Input: part model. Units: mm. Frame: model coordinates. A direction names the side the tool comes from. Coordinates: 2 decimals unless noted, no trailing zeros. Order: outer loops, then holes, each group sorted by start corner. A loop starts at its lowest first (then second) coordinate and runs counter-clockwise, first axis right, second up. Notation, with made-up numbers: (1, 16.5) -> (9, 16.5) arc R14 cw to (9, 20.5) -> close; hole circle Ø4 at (-35, -7.5). An arc over 180 degrees is marked (long way). One line per question, with ' | ' between items.
```python
from build123d import *

# Parameters (mm, degrees)
SKETCH1_W           = 50
SKETCH1_H           = 60
BOSS_EXTRUDE1_DEPTH = 2.85
SKETCH2_W           = 10
SKETCH2_H           = 2.85
BOSS_EXTRUDE2_DEPTH = 2.85
CUT_EXTRUDE1_DEPTH  = 42.379282256
SKETCH4_R           = 1.425
SKETCH4_W           = 10
SKETCH4_H           = 2.85
CUT_EXTRUDE2_DEPTH  = 42.379282256


with BuildPart() as part:
    # Sketch1 → Boss-Extrude1 (new body)
    with BuildSketch(Plane(origin=(0, 0, 0), x_dir=(1, 0, 0), z_dir=(0, 1, 0))):
        Rectangle(SKETCH1_W, SKETCH1_H)
    extrude(amount=BOSS_EXTRUDE1_DEPTH)

    # Sketch2 → Boss-Extrude2 (add)
    with BuildSketch(Plane(origin=(0, 2.85, 0), x_dir=(1, 0, 0), z_dir=(0, 1, 0))):
        with Locations((-15, 31.425)):
            Rectangle(SKETCH2_W, SKETCH2_H)
        with Locations((15, 31.425)):
            Rectangle(SKETCH2_W, SKETCH2_H)
    boss_extrude2 = extrude(amount=-BOSS_EXTRUDE2_DEPTH)

    # Sketch3 → Cut-Extrude1 (cut, through all)
    with BuildSketch(Plane(origin=(0, 2.85, 0), x_dir=(1, 0, 0), z_dir=(0, 1, 0))):
        Polygon((-4, 26), (-1.7, 26), (-1.7, 30), (1.7, 30), (1.7, 26), (4, 26), (4, 23), (1.7, 23), (1.7, 20), (-1.7, 20), (-1.7, 23), (-4, 23), align=None)
    cut_extrude1 = extrude(amount=-CUT_EXTRUDE1_DEPTH, mode=Mode.SUBTRACT)

    # Mirror1: Boss-Extrude2, Cut-Extrude1 across plane
    add(boss_extrude2.mirror(Plane.XY))
    add(cut_extrude1.mirror(Plane.XY), mode=Mode.SUBTRACT)

    # Sketch4 → Cut-Extrude2 (cut, through all)
    with BuildSketch(Plane(origin=(0, 2.85, 0), x_dir=(1, 0, 0), z_dir=(0, 1, 0))):
        with Locations(Location((0, 0.515, 0), (0, 0, 270))):
            Circle(SKETCH4_R)
        with Locations((-15, 0.515)):
            Rectangle(SKETCH4_W, SKETCH4_H)
        with Locations((15, 0.515)):
            Rectangle(SKETCH4_W, SKETCH4_H)
    extrude(amount=-CUT_EXTRUDE2_DEPTH, mode=Mode.SUBTRACT)


solid = part.part
```
1. Cut plane B-B, the plane z = -21. Return loops of the section in (x, y).
Recorded:
outline: (-25, 0) -> (-1.7, 0) -> (-1.7, 2.85) -> (-25, 2.85) -> close; (1.7, 0) -> (25, 0) -> (25, 2.85) -> (1.7, 2.85) -> close
2. Cut plane D-D, the plane y = 0.9. State how many separate pieces and enclosed holes the cut face has, and give its area (3 significant figures).
Recorded:
separate pieces: 1 | enclosed holes: 3 | area: 2,960 mm^2
3. Mould query, pull axis X, two halves, no side actions, for faces 6 (the face through (-20, 1, 31)), 7 (the face through (-1.7, 1, -28)), 8 (the face through (25, 1, 0)), 9 (the face through (15, 1, 32.85)). Classes: released by +X, released by -X, zero draft, split by the parting line, or undercut.
Recorded:
face 6: released by -X | face 7: undercut | face 8: released by +X | face 9: zero draft
4. Cut plane C-C, the plane z = -1. Return loops of the section in (x, y), and give its area (3 significant figures).
Recorded:
outline: (-25, 0) -> (-20, 0) -> (-20, 2.85) -> (-25, 2.85) -> close; (-10, 0) -> (-1.34, 0) -> (-1.34, 2.85) -> (-10, 2.85) -> close; (1.34, 0) -> (10, 0) -> (10, 2.85) -> (1.34, 2.85) -> close; (20, 0) -> (25, 0) -> (25, 2.85) -> (20, 2.85) -> close | area: 77.9 mm^2
5. Pin query (flat end, axial travel): pin 1 Ø1.2 at (x, y) = (3, 1.5) entering from -Z; pin 2 Ø0.9 at (y, z) = (2, 32) entering from -X; pin 3 Ø0.9 at (x, y) = (0.5, 1.5) entering from -Z. Return the tip coordinate at first contact, or that it passes through.
Recorded:
pin 1: stops at z = -30 | pin 2: stops at x = -20 | pin 3: stops at z = -20
6. Access query for faces 1 (the face through (-25, 1, 0)), 2 (the face through (-20, 1, 0)), 3 (the face through (-20, 1, -31)), 4 (the face through (1.7, 1, -22)), 5 (the face through (0, 1, 20)). Directions: +Z, -Z, +X, -X, +Y, -Y. A direction counts if a zero-diameter tool reaches every point of the face in a straight line with its end or side. Return the directions, or none.
Recorded:
face 1: +Z, -Z, -X, +Y, -Y | face 2: +Y, -Y | face 3: -Z, -X, +Y, -Y | face 4: -Z, +Y, -Y | face 5: +Z, +Y, -Y
7. Cut plane A-A, the plane x = 0. Return loops of the section in (y, z).
Recorded:
outline: (0, -20) -> (2.85, -20) -> (2.85, -1.94) -> (0, -1.94) -> close; (0, 0.91) -> (2.85, 0.91) -> (2.85, 20) -> (0, 20) -> close
8. Ray query, line 1 (Z direction, x = -2, y = 0.7); line 2 (X direction, y = 0.25, z = 24); line 3 (Z direction, x = -16, y = 2.65). Return the intervals inside material, ascending. Write a range as [from, to].
Recorded:
line 1: z = [-30, -26], [-23, 23], [26, 30] | line 2: x = [-25, -4], [4, 25] | line 3: z = [-32.85, -1.94], [0.91, 32.85]
